```python
from build123d import *

# Parameters (mm, degrees)
SKETCH_1_R      = 5
EXTRUDE_1_DEPTH = 1


with BuildPart() as part:
    # 草图1 → 凸台-拉伸1 (new body)
    with BuildSketch(Plane.XY):
        Circle(SKETCH_1_R)
        with BuildLine():
            Line((-0.318380039, -1.005793851), (1.720384349, -1.005793851))
            Line((1.720384349, -1.005793851), (1.788940866, -1.005793851))
            Line((1.788940866, -1.005793851), (2.645033635, -3.640576475))
            Line((2.645033635, -3.640576475), (0, -1.718847051))
            Line((0, -1.718847051), (-2.645033635, -3.640576475))
            Line((-2.645033635, -3.640576475), (-1.788940866, -1.005793851))
            Line((-1.788940866, -1.005793851), (-1.252770646, -1.005793851))
            Line((-1.252770646, -1.005793851), (-1.252770646, -0.94707964))
            ThreePointArc((-1.252770646, -0.94707964), (-1.24398385, -0.925866437), (-1.222770646, -0.91707964))
            Line((-1.222770646, -0.91707964), (-1.054612311, -0.91707964))
            Line((-1.054612311, -0.91707964), (-0.9619207, -0.552326205))
            Line((-0.9619207, -0.552326205), (-0.904349803, -0.552326205))
            ThreePointArc((-0.904349803, -0.552326205), (-0.8831366, -0.561113001), (-0.874349803, -0.582326205))
            Line((-0.874349803, -0.582326205), (-0.874349803, -0.641189165))
            Line((-0.874349803, -0.641189165), (-0.466949327, -0.91707964))
            Line((-0.466949327, -0.91707964), (-0.348380039, -0.91707964))
            ThreePointArc((-0.348380039, -0.91707964), (-0.327166836, -0.925866437), (-0.318380039, -0.94707964))
            Line((-0.318380039, -0.94707964), (-0.318380039, -1.005793851))
        make_face(mode=Mode.SUBTRACT)
        with BuildLine():
            add(Edge.make_bspline(
                [(-1.842127605, 0.722748563), (-1.53406941, -0.398381027), (0.099478664, -1.328305568), (1.067230007, -0.372749727)],
                knots=[0, 0, 0, 0, 1, 1, 1, 1], degree=3))
            add(Edge.make_bspline(
                [(-1.842127605, 0.722748563), (-1.393572664, -0.207863674), (0.098677528, -1.088124965), (1.067230007, -0.372749727)],
                knots=[0, 0, 0, 0, 1, 1, 1, 1], degree=3))
        make_face(mode=Mode.SUBTRACT)
        with BuildLine():
            add(Edge.make_bspline(
                [(-1.502914254, 0.514806758), (-0.935681631, -0.359051857), (0.725669726, -1.040375739), (1.416769627, 0.071599659)],
                knots=[0, 0, 0, 0, 1, 1, 1, 1], degree=3))
            add(Edge.make_bspline(
                [(-1.502914254, 0.514806758), (-0.839650751, -0.216239781), (0.600989178, -0.75455265), (1.416769627, 0.071599659)],
                knots=[0, 0, 0, 0, 1, 1, 1, 1], degree=3))
        make_face(mode=Mode.SUBTRACT)
        with BuildLine():
            add(Edge.make_bspline(
                [(-1.089784914, 0.404626073), (-0.465343338, -0.314626601), (1.155887368, -0.588128356), (1.526429115, 0.514806758)],
                knots=[0, 0, 0, 0, 1, 1, 1, 1], degree=3))
            add(Edge.make_bspline(
                [(-1.089784914, 0.404626073), (-0.382266231, -0.142810276), (0.950686118, -0.345522278), (1.526429115, 0.514806758)],
                knots=[0, 0, 0, 0, 1, 1, 1, 1], degree=3))
        make_face(mode=Mode.SUBTRACT)
        Polygon((-4.279754323, 1.390576475), (-2.15, 1.390576475), (-2.15, -0.066596805), (-2.15, -0.156780615), align=None, mode=Mode.SUBTRACT)
        Polygon((-1.010312947, 1.390576475), (0, 4.5), (1.010312947, 1.390576475), align=None, mode=Mode.SUBTRACT)
        with BuildLine():
            add(Edge.make_bspline(
                [(-0.725576796, 0.369276137), (-0.035664287, -0.02834489), (1.378252258, -0.188638059), (1.489870248, 0.924289378)],
                knots=[0, 0, 0, 0, 1, 1, 1, 1], degree=3))
            add(Edge.make_bspline(
                [(-0.725576796, 0.369276137), (-0.039042271, 0.197569955), (1.170700763, -0.001897128), (1.489870248, 0.924289378)],
                knots=[0, 0, 0, 0, 1, 1, 1, 1], degree=3))
        make_face(mode=Mode.SUBTRACT)
        with BuildLine():
            ThreePointArc((-0.712399817, 0.947220378), (-0.736081707, 0.958803862), (-0.741475678, 0.984609173))
            Line((-0.741475678, 0.984609173), (-0.7280269, 1.03753185))
            ThreePointArc((-0.7280269, 1.03753185), (-0.717367555, 1.053824945), (-0.698951039, 1.060143055))
            Line((-0.698951039, 1.060143055), (0.76839361, 1.060143055))
            ThreePointArc((0.76839361, 1.060143055), (0.805059277, 1.044137597), (0.818250912, 1.00636821))
            Line((0.818250912, 1.00636821), (0.774791122, 0.432361166))
            ThreePointArc((0.774791122, 0.432361166), (0.765273466, 0.412626673), (0.744876741, 0.404626073))
            Line((0.744876741, 0.404626073), (0.626290225, 0.404626073))
            ThreePointArc((0.626290225, 0.404626073), (0.604290825, 0.414229348), (0.596375844, 0.43689098))
            Line((0.596375844, 0.43689098), (0.610235616, 0.61994771))
            ThreePointArc((0.610235616, 0.61994771), (0.53231079, 0.847272593), (0.313771729, 0.947220378))
            Line((0.313771729, 0.947220378), (0.006808985, 0.947220378))
            Line((0.006808985, 0.947220378), (-0.131834864, 0.401638961))
            ThreePointArc((-0.131834864, 0.401638961), (-0.144081452, 0.38419279), (-0.164823975, 0.379284077))
            Line((-0.164823975, 0.379284077), (-0.673570673, 0.446217721))
            ThreePointArc((-0.673570673, 0.446217721), (-0.694492389, 0.459132127), (-0.698733285, 0.483350196))
            Line((-0.698733285, 0.483350196), (-0.580853999, 0.947220378))
            Line((-0.580853999, 0.947220378), (-0.712399817, 0.947220378))
        make_face(mode=Mode.SUBTRACT)
        Polygon((4.279754323, 1.390576475), (2, -0.265761995), (2, -0.022653284), (2, 1.390576475), align=None, mode=Mode.SUBTRACT)
    extrude(amount=EXTRUDE_1_DEPTH)


solid = part.part
```
Could you check a few things on this model? Use its own coordinates, in mm. A direction names the side the tool comes from. Round coordinates to 2 decimals unless told otherwise and drop trailing zeros. Loops run counter-clockwise (first coordinate to the right, second up) from the corner with the lowest first, then second, coordinate; pieces in that order, holes last. Notation, with made-up numbers: (31, -3.75) - (37, -3.75) arc R5 cw to (37, 4.25) - close; hole circle Ø1 at (61.5, -25). An arc over 180 degrees is marked (long way). Answer as CSV lines item,"result".
1. Please list where these lines run through material, in increasing order: line 1 along X through (y, z) = (-2, 0.3); line 2 along X through (y, z) = (-2.75, 0.95); line 3 along Y through (x, z) = (-3.75, 0.6). Write a range as [from, to].
Filled in:
line 1,"x = [-4.58, -2.11], [-0.39, 0.39], [2.11, 4.58]"
line 2,"x = [-4.18, -2.36], [-1.42, 1.42], [2.36, 4.18]"
line 3,"y = [-3.31, 1.01], [1.39, 3.31]"
2. On a 3-axis mill with a long thin cutter (end or side, diameter ignored), from which of +Z, -Z, +X, -X, +Y, -Y can I reach the whole of each face in a straight line? I mean faces 4 (the face through (3.156, 0.574, 0.493)), 5 (the face through (1, 1, 0)). Say none if no direction works.
Filled in:
face 4,"+Z, -Z"
face 5,"-Z, +X, -X, +Y, -Y"
3. We'd pull the mould along X, two halves only. Please class faces 1 (the face through (3.1, 1.391, 0.5)), 2 (the face through (1, 1, 1)), 3 (the face through (-1.08, -4.88, 0.49)): +X half, -X half, draft (parallel to the pull), parting line (faces both ways), or undercut.
Filled in:
face 1,"undercut"
face 2,"draft"
face 3,"parting line"
4. I want a section at B-B on y = -2.5. List the corners of the cut face in (x, z) for me, then the cut area to 3 significant figures.
Filled in:
outline,"(-4.33, 0) - (-2.27, 0) - (-2.27, 1) - (-4.33, 1) - close; (-1.08, 0) - (1.08, 0) - (1.08, 1) - (-1.08, 1) - close; (2.27, 0) - (4.33, 0) - (4.33, 1) - (2.27, 1) - close"
area,"6.26 mm^2"
5. I want a section at C-C on y = 3.5. List the corners of the cut face in (x, z) for me.
Filled in:
outline,"(-3.57, 0) - (-0.32, 0) - (-0.32, 1) - (-3.57, 1) - close; (0.32, 0) - (3.57, 0) - (3.57, 1) - (0.32, 1) - close"
6. I want a section at D-D on z = 0.45. Count the separate pieces of the cut face and the enclosed holes in it, then the cut area to 3 significant figures.
Filled in:
separate pieces,"1"
enclosed holes,"9"
area,"63.1 mm^2"
7. I want a section at A-A on y = 2. List the corners of the cut face in (x, z) for me, then the cut area to 3 significant figures.
Filled in:
outline,"(-4.58, 0) - (-0.81, 0) - (-0.81, 1) - (-4.58, 1) - close; (0.81, 0) - (4.58, 0) - (4.58, 1) - (0.81, 1) - close"
area,"7.54 mm^2"
